The listing builds one solid part. Answer for the finished solid, in the listing's coordinates (mm). Face numbers are marked on the shaded views. A direction names the side the tool comes from. Give positions to 0.01 mm unless a question says otherwise; leave off trailing zeros. Loops run counter-clockwise (first coordinate to the right, second up) from the corner with the lowest first, then second, coordinate; pieces in that order, holes last. Notation, with made-up numbers: (-31, 88) - (25, 88) arc R24 cw to (25, 114) - close; hole circle Ø4 at (26, 49). An arc over 180 degrees is marked (long way). Answer as CSV lines item,"result". Start each with the question number.
1) A cutting plane is placed at B-B (z = 14). Determine the outline of the cut face in (x, y).
2) Flat-ended cylindrical pins translate along their axes: pin 1 (4 mm diameter, centred on x = 146.5, y = 14, fed in from +Z); pin 2 (1.5 mm diameter, centred on x = 133.5, y = -4.5, fed in from +Z); pin 3 (3 mm diameter, centred on x = 122.5, z = -2.5, fed in from +Y). Find the tip coordinate at first contact, or state that the pin passes through.
3) A cutting plane is placed at A-A (x = 94). Determine the outline of the cut face in (y, z).
4) Find the intervals of material crossed by line 1 along Y through (x, z) = (-2.25, 0); line 2 along X through (y, z) = (-12.5, -22), in increasing order.
5) For the marked faces 1 and 2, determine the directions among +Z, -Z, +X, -X, +Y, -Y from which every point of the face is accessible in a straight line to the end or side of a thin tool.
```python
from build123d import *

# Parameters (mm, degrees)
HOLE1_D           = 9.73836
HOLE1_DEPTH       = 28.062477616
HOLE1_CSINK_D     = 11.1125
HOLE1_CSINK_ANGLE = 90
HOLE1_TIP         = 2.811222384


with BuildPart() as part:
    # Sketch1 → Revolve1 (revolve)
    with BuildSketch(Plane.XY):
        Polygon((-22.225, 0), (-22.225, 8.001), (145.3642, 8.001), (145.3642, 25.4508), (173.8376, 25.4508), (173.8376, 0), align=None)
    revolve(axis=Axis((173.8376, 0, 0), (-1, 0, 0)))

    # Hole1
    with Locations(Plane.ZY.offset(22.225)):
        with Locations((0, 0)):
            CounterSinkHole(HOLE1_D / 2, HOLE1_CSINK_D / 2, depth=HOLE1_DEPTH, counter_sink_angle=HOLE1_CSINK_ANGLE)
            with Locations((0, 0, -(HOLE1_DEPTH + HOLE1_TIP / 2))):  # 120° drill point
                Cone(0, HOLE1_D / 2, HOLE1_TIP, mode=Mode.SUBTRACT)


solid = part.part
```
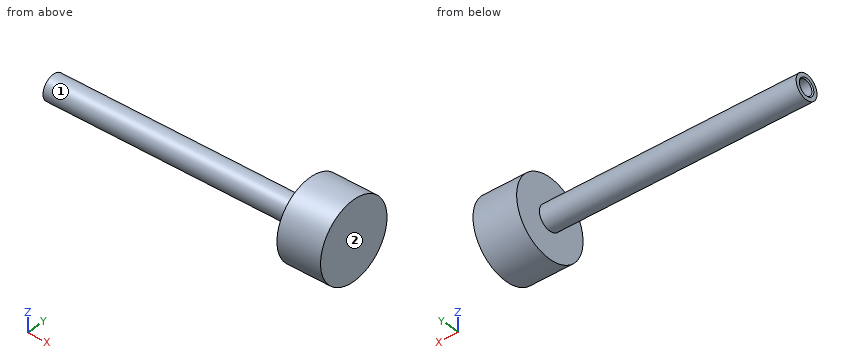
Ans:
1,outline,"(145.36, -21.25) - (173.84, -21.25) - (173.84, 21.25) - (145.36, 21.25) - close"
2,pin 1,"z = 22.44"
2,pin 2,"z = 7.07"
2,pin 3,"y = 7.94"
3,outline,"circle Ø16 at (0, 0)"
4,line 1,"-8 to -4.87, 4.87 to 8"
4,line 2,"145.36 to 173.84"
5,face 1,"-X"
5,face 2,"+Z, -Z, +X, +Y, -Y"
